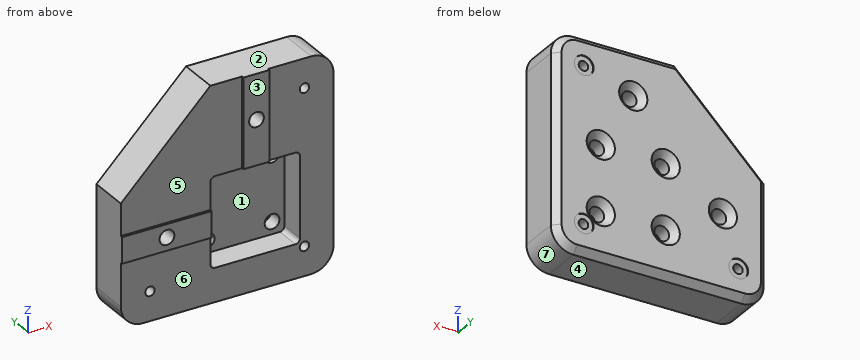
```python
from build123d import *

# Parameters (mm, degrees)
SKETCH_1_W                 = 80
SKETCH_1_H                 = 80
EXTRUDE_314_DEPTH          = 21
EXTRUDE_603_DEPTH          = 21
CUT_EXTRUDE_830_DEPTH      = 81.566742518
SKETCH_3_W                 = 40
SKETCH_3_H                 = 40
CUT_EXTRUDE_1062_DEPTH     = 11.5
FILLET_1_R                 = 2
SKETCH_14_W                = 40
SKETCH_14_H                = 11.6
SKETCH_14_W_2              = 11.6
SKETCH_14_H_2              = 40
EXTRUDE_1761_DEPTH         = 1
HOLE_WIZARD_M6_D           = 6.6
HOLE_WIZARD_M6_CSINK_D     = 12.6
HOLE_WIZARD_M6_CSINK_ANGLE = 90
HOLE_WIZARD_M5_D           = 4.2
HOLE_WIZARD_M5_CSINK_D     = 5.05
HOLE_WIZARD_M5_CSINK_ANGLE = 90
FILLET_2_R                 = 10
CHAMFER_1_SIZE             = 3
SKETCH_15_R                = 4.3
CUT_EXTRUDE_1_DEPTH        = 0.4


with BuildPart() as part:
    # Эскиз1 → Extrude 314 (new body)
    with BuildSketch(Plane(origin=(0, 0, 0), x_dir=(1, 0, 0), z_dir=(0, 1, 0))):
        Rectangle(SKETCH_1_W, SKETCH_1_H)
    extrude(amount=EXTRUDE_314_DEPTH)

    # Эскиз11 → Extrude 603 (add)
    with BuildSketch(Plane(origin=(0, 21, 0), x_dir=(1, 0, 0), z_dir=(0, 1, 0))):
        Polygon((40, -40), (55, -40), (55, 55), (-40, 55), (-40, 40), (40, 40), align=None)
    extrude(amount=-EXTRUDE_603_DEPTH)

    # Эскиз2 → Cut-Extrude 830 (cut, through all)
    with BuildSketch(Plane(origin=(0, 21, 0), x_dir=(1, 0, 0), z_dir=(0, 1, 0))):
        Polygon((-40, -40), (-40, 0), (0, -40), align=None)
    extrude(amount=-CUT_EXTRUDE_830_DEPTH, mode=Mode.SUBTRACT)

    # Эскиз3 → Cut-Extrude 1062 (cut)
    with BuildSketch(Plane.XZ):
        with Locations((20, -20)):
            Rectangle(SKETCH_3_W, SKETCH_3_H)
    extrude(amount=-CUT_EXTRUDE_1062_DEPTH, mode=Mode.SUBTRACT)

    # Скругление1
    fillet_1_edges = [part.edges().sort_by_distance(p)[0] for p in [
        (40, 5.75, 0),
        (40, 5.75, -40),
        (0, 5.75, -40),
        (0, 5.75, 0),
    ]]
    fillet(fillet_1_edges, radius=FILLET_1_R)

    # Эскиз14 → Extrude 1761 (add)
    with BuildSketch(Plane.XZ):
        with Locations((-20, -20)):
            Rectangle(SKETCH_14_W, SKETCH_14_H)
        with Locations((20, 20)):
            Rectangle(SKETCH_14_W_2, SKETCH_14_H_2)
    extrude(amount=EXTRUDE_1761_DEPTH)

    # Крепление-M6 (through all)
    with Locations(Plane(origin=(0, 21, 0), x_dir=(1, 0, 0), z_dir=(0, 1, 0))):
        with Locations((-20, 20), (20, -20), (5.5, 34.5), (34.5, 34.5), (34.5, 5.5), (5.5, 5.5)):
            CounterSinkHole(HOLE_WIZARD_M6_D / 2, HOLE_WIZARD_M6_CSINK_D / 2, counter_sink_angle=HOLE_WIZARD_M6_CSINK_ANGLE)

    # Шкивы-M5 (through all)
    with Locations(Plane(origin=(0, 21, 0), x_dir=(1, 0, 0), z_dir=(0, 1, 0))):
        with Locations((42, 42), (-27, 42), (42, -27)):
            CounterSinkHole(HOLE_WIZARD_M5_D / 2, HOLE_WIZARD_M5_CSINK_D / 2, counter_sink_angle=HOLE_WIZARD_M5_CSINK_ANGLE)

    # Скругление2
    fillet_2_edges = [part.edges().sort_by_distance(p)[0] for p in [
        (-40, 10.5, -55),
        (55, 10.5, -55),
        (55, 10.5, 40),
    ]]
    fillet(fillet_2_edges, radius=FILLET_2_R)

    # Фаска1
    chamfer_1_edges = [part.edges().sort_by_distance(p)[0] for p in [
        (7.5, 21, -55),
        (55, 21, -7.5),
        (-40, 21, -22.5),
        (52.071067812, 21, 37.071067812),
        (52.071067812, 21, -52.071067812),
        (-37.071067812, 21, -52.071067812),
        (22.5, 21, 40),
        (-20, 21, 20),
    ]]
    chamfer(chamfer_1_edges, length=CHAMFER_1_SIZE)

    # Эскиз15 → Вырез-Вытянуть1 (cut)
    with BuildSketch(Plane(origin=(0, 21, 0), x_dir=(1, 0, 0), z_dir=(0, 1, 0))):
        with Locations(Location((42, 42, 0), (0, 0, 270))):
            Circle(SKETCH_15_R)
        with Locations(Location((-27, 42, 0), (0, 0, 270))):
            Circle(SKETCH_15_R)
        with Locations(Location((42, -27, 0), (0, 0, 270))):
            Circle(SKETCH_15_R)
    extrude(amount=-CUT_EXTRUDE_1_DEPTH, mode=Mode.SUBTRACT)


solid = part.part
```
Part model, mm, in its own coordinate system. Face numbers are marked on the shaded views. A direction names the side the tool comes from. Coordinates: 2 decimals unless noted, no trailing zeros. Loops run counter-clockwise (first coordinate to the right, second up) from the corner with the lowest first, then second, coordinate; pieces in that order, holes last. Notation, with made-up numbers: (54.25, 40) - (102.25, 40) arc R18 ccw to (102.25, 72) - close; hole circle Ø3 at (57.5, -20). An arc over 180 degrees is marked (long way). Write item = value, one per line. Start each with the question number.
Item 1: Cut at A-A, the plane x = 42. Give the cut face in (y, z) (3 decimals).
Item 2: Cut at C-C, the plane y = 9.75. Give the cut face in (x, z), and give its area (3 significant figures).
Item 3: Mould opens along Z. For the marked faces 1, 2, 3 and 4 say: released by +Z, released by -Z, zero draft, split by the parting line, or undercut.
Item 4: Cut at D-D, the plane x = 20. Give the cut face in (y, z).
Item 5: Flat gauge pins, fed straight in: pin 1 Ø5 at (x, z) = (11, -7.5) entering from +Y; pin 2 Ø7 at (x, z) = (-27, -42) entering from -Y; pin 3 Ø6.5 at (x, z) = (42, 27) entering from +Y; pin 4 Ø5 at (x, y) = (-12, 10) entering from +Z. Where does each tip first touch, or does it go through?
Item 6: Cut at B-B, the plane z = -5.5. Give the cut face in (x, y).
Item 7: 3-axis set-ups, long thin cutter, end or side, ignore diameter. For the marked faces 5, 6 and 7: which of +Z, -Z, +X, -X, +Y, -Y reach the whole face in a straight line?
Item 8: Wall check: L1, parallel to Z at x = 34.5, y = 14; L2, parallel to X at y = 9.75, z = -20; L3, parallel to X at y = 1.5, z = -33. Give the ranges that are in metal, low to high. Write a range as from..to.
The answers:
q1.outline = (0, -55) - (18, -55) - (21, -52) - (21, -46.3) - (20.6, -46.3) - (20.6, -44.125) - (20.575, -44.1) - (0, -44.1) - close; (0, -39.9) - (20.575, -39.9) - (20.6, -39.875) - (20.6, -37.7) - (21, -37.7) - (21, 22.7) - (20.6, 22.7) - (20.6, 24.875) - (20.575, 24.9) - (0, 24.9) - close; (0, 29.1) - (20.575, 29.1) - (20.6, 29.125) - (20.6, 31.3) - (21, 31.3) - (21, 37) - (18, 40) - (0, 40) - close
q2.outline = (-40, -45) arc R10 ccw to (-30, -55) - (45, -55) arc R10 ccw to (55, -45) - (55, 30) arc R10 ccw to (45, 40) - (0, 40) - (-40, 0) - close; hole circle Ø4.2 at (-27, -42); hole circle Ø6.6 at (-20, -20); hole (0, -38) arc R2 ccw to (2, -40) - (38, -40) arc R2 ccw to (40, -38) - (40, -2) arc R2 ccw to (38, 0) - (2, 0) arc R2 ccw to (0, -2) - close; hole circle Ø6.6 at (20, 20); hole circle Ø4.2 at (42, -42); hole circle Ø4.2 at (42, 27)
q2.area = 6,450 mm2
q3.face_1 = undercut
q3.face_2 = released by +Z
q3.face_3 = zero draft
q3.face_4 = released by -Z
q4.outline = (-1, 0) - (11.5, 0) - (11.5, -40) - (0, -40) - (0, -55) - (18, -55) - (21, -52) - (21, 13.7) - (18, 16.7) - (-1, 16.7) - close; (-1, 23.3) - (18, 23.3) - (21, 26.3) - (21, 37) - (18, 40) - (-1, 40) - close
q5.pin_1 = 21
q5.pin_2 = 0
q5.pin_3 = 20.6
q5.pin_4 = 30.5
q6.outline = (-40, 0) - (0, 0) - (0, 11.5) - (2.2, 11.5) - (2.2, 18) - (-0.8, 21) - (-37, 21) - (-40, 18) - close; (8.8, 11.5) - (31.2, 11.5) - (31.2, 18) - (28.2, 21) - (11.8, 21) - (8.8, 18) - close; (37.8, 11.5) - (40, 11.5) - (40, 0) - (55, 0) - (55, 18) - (52, 21) - (40.8, 21) - (37.8, 18) - close
q7.face_5 = +Z, -X, -Y
q7.face_6 = -Z, +X, -Y
q7.face_7 = -Z, +X, +Y, -Y
q8.L1 = -55..-37.8, -31.2..-8.8, -2.2..40
q8.L2 = -40..-23.3, -16.7..0, 40..55
q8.L3 = -40..0, 40..55
